Geometry: final body of the model. Coordinates: model frame, mm. Give positions to 0.01 mm unless a question says otherwise; leave off trailing zeros. Write each loop counter-clockwise with the first axis right and the second up, starting at its lowest first coordinate (ties: lowest second). Pieces come first, ordered by that corner, then holes. Notation, with made-up numbers: M -0.75,-34 L 58.25,-34 A9 cw 58.25,-26 Z; hole C 62.25,87.5 d7. An arc over 180 degrees is marked long. Use a Markdown table: item, result. Add a question column.
(1) Material intervals for L1, parallel to X at y = -19, z = 0.6; L2, parallel to Y at x = 0.5, z = 0.65; L3, parallel to Y at x = 5.5, z = 0.4, sorted ascending.
(2) Cut plane C-C (z = 0.8). State how many separate pieces and enclosed holes the cut face has, plus the area to 3 significant figures.
(3) Cut plane A-A (y = -25.5). Output: boundary loops of the cut face in (x, z).
(4) Cut plane B-B (x = 0). Output: boundary loops of the cut face in (y, z).
(5) Pin query (flat end, axial travel): pin 1 Ø4 at (x, y) = (22.08, 12.75) entering from -Z. Return the tip coordinate at first contact, or that it passes through.
(6) Cut plane D-D (y = -19.5). Output: boundary loops of the cut face in (x, z), plus the area to 3 significant figures.
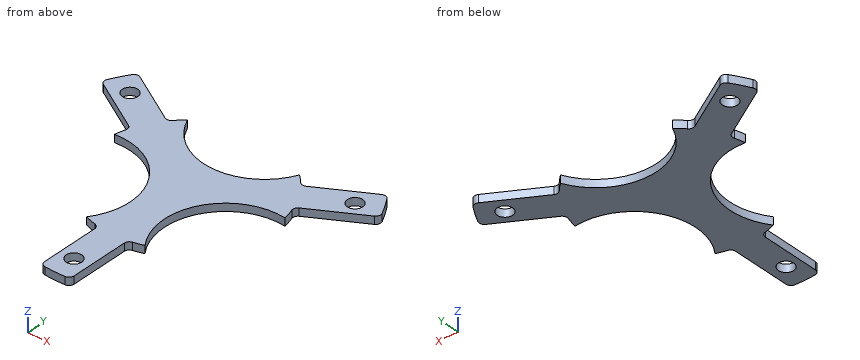
```python
from build123d import *

# Parameters (mm, degrees)
F0_R     = 1.5
F1_DEPTH = 1.5


with BuildPart() as f1:
    # F0 (on Top) → F1 (new body)
    with BuildSketch(Plane.XY):
        with BuildLine():
            ThreePointArc((-23.679947, 16.87634), (-24.409064, 16.983713), (-25.013738, 16.562394))
            ThreePointArc((-25.013738, 16.562394), (-26.038785, 14.899049), (-26.953386, 13.172509))
            ThreePointArc((-26.953386, 13.172509), (-27.01136, 12.441433), (-26.55494, 11.8674))
            Line((-26.55494, 11.8674), (-16.698684, 6.176888))
            ThreePointArc((-16.698684, 6.176888), (-16.267754, 5.676061), (-16.243202, 5.015815))
            ThreePointArc((-16.243202, 5.015815), (-16.513498, 4.037868), (-16.724972, 3.045539))
            ThreePointArc((-16.724972, 3.045539), (-4.985979, -2.878656), (-5.724972, -16.00702))
            ThreePointArc((-5.724972, -16.00702), (-4.655459, -16.350129), (-3.565623, -16.621863))
            ThreePointArc((-3.565623, -16.621863), (-2.997631, -16.971027), (-2.775366, -17.59962))
            Line((-2.775366, -17.59962), (-2.775366, -28.945605))
            ThreePointArc((-2.775366, -28.945605), (-2.503795, -29.630726), (-1.836585, -29.94373))
            ThreePointArc((-1.836585, -29.94373), (0.116437, -29.999774), (2.068966, -29.928571))
            ThreePointArc((2.068966, -29.928571), (2.731083, -29.613241), (3, -28.930952))
            Line((3, -28.930952), (3, -17.549929))
            ThreePointArc((3, -17.549929), (3.218264, -16.926319), (3.777778, -16.574933))
            ThreePointArc((3.777778, -16.574933), (4.759852, -16.320043), (5.724972, -16.00702))
            ThreePointArc((5.724972, -16.00702), (4.985979, -2.878656), (16.724972, 3.045539))
            ThreePointArc((16.724972, 3.045539), (16.487356, 4.143319), (16.177767, 5.223011))
            ThreePointArc((16.177767, 5.223011), (16.196156, 5.889489), (16.629401, 6.396273))
            Line((16.629401, 6.396273), (26.455312, 12.069266))
            ThreePointArc((26.455312, 12.069266), (26.912859, 12.647013), (26.850323, 13.381336))
            ThreePointArc((26.850323, 13.381336), (25.922348, 15.100725), (24.88442, 16.756062))
            ThreePointArc((24.88442, 16.756062), (24.280277, 17.171808), (23.55494, 17.063552))
            Line((23.55494, 17.063552), (13.698684, 11.373041))
            ThreePointArc((13.698684, 11.373041), (13.04949, 11.250258), (12.465424, 11.559118))
            ThreePointArc((12.465424, 11.559118), (11.753646, 12.282175), (11, 12.961481))
            ThreePointArc((11, 12.961481), (0, 5.757313), (-11, 12.961481))
            ThreePointArc((-11, 12.961481), (-11.831897, 12.20681), (-12.612144, 11.398852))
            ThreePointArc((-12.612144, 11.398852), (-13.198525, 11.081538), (-13.854035, 11.203347))
            Line((-13.854035, 11.203347), (-23.679947, 16.87634))
        make_face()
        with Locations((0, -25.5)):
            Circle(F0_R, mode=Mode.SUBTRACT)
        with Locations((-22.083648, 12.75)):
            Circle(F0_R, mode=Mode.SUBTRACT)
        with Locations((22.083648, 12.75)):
            Circle(F0_R, mode=Mode.SUBTRACT)
    extrude(amount=F1_DEPTH)


solid = f1.part
```
Answer list:
| question | item | result |
|---|---|---|
| 1 | L1 | -2.78 to 3 |
| 1 | L2 | -30 to -26.91, -24.09 to 5.77 |
| 1 | L3 | -16.09 to -15.69, -2.07 to 7.09 |
| 2 | separate pieces | 1 |
| 2 | enclosed holes | 3 |
| 2 | area | 587 mm² |
| 3 | outline | M -2.78,0 L -1.5,0 L -1.5,1.5 L -2.78,1.5 Z; M 1.5,0 L 3,0 L 3,1.5 L 1.5,1.5 Z |
| 4 | outline | M -30,0 L -27,0 L -27,1.5 L -30,1.5 Z; M -24,0 L 5.76,0 L 5.76,1.5 L -24,1.5 Z |
| 5 | pin 1 | z = 0 |
| 6 | outline | M -2.78,0 L 3,0 L 3,1.5 L -2.78,1.5 Z |
| 6 | area | 8.66 mm² |
